Geometry: final body of the model. Coordinates: model frame, mm. Face numbers are marked on the shaded views. Coordinates: 2 decimals unless noted, no trailing zeros. Loops run counter-clockwise (first coordinate to the right, second up) from the corner with the lowest first, then second, coordinate; pieces in that order, holes last. Notation, with made-up numbers: (-24.5, -13.75) - (14.5, -13.75) arc R16 cw to (14.5, -3.75) - close; hole circle Ø9 at (75.25, 24.5). An arc over 180 degrees is marked (long way). Return JSON: item names as keys, results as strings.
from build123d import *

# Parameters (mm, degrees)
ESQUISSE1_W               = 58
ESQUISSE1_H               = 65
T_LE_DE_BASE_PLI_E1_DEPTH = 3
ENL_V_MAT_EXTRU_1_REACH   = 45.661
ESQUISSE6_R               = 2
ENL_V_MAT_EXTRU_2_REACH   = 45.661
ESQUISSE7_R               = 2
ESQUISSE8_R               = 4
ESQUISSE8_R_2             = 2
BOSS_EXTRU_1_DEPTH        = 2.7
ESQUISSE11_R              = 4
BOSS_EXTRU_3_DEPTH        = 1
ENL_V_MAT_EXTRU_3_REACH   = 46.07
ESQUISSE9_W               = 40
ESQUISSE9_H               = 34
ESQUISSE12_R              = 4
ESQUISSE12_R_2            = 2
BOSS_EXTRU_4_DEPTH        = 3.7
ESQUISSE13_R              = 2
BOSS_EXTRU_5_DEPTH        = 1


# Sheet-metal steps are written as plain solids
with BuildPart() as part:
    # Esquisse1 → Tôle de base pliée1 (new body)
    with BuildSketch(Plane.XY):
        Rectangle(ESQUISSE1_W, ESQUISSE1_H)
    extrude(amount=-T_LE_DE_BASE_PLI_E1_DEPTH)

    # Esquisse6 → Enlèv. mat.-Extru.1 (cut, up to next)
    with BuildSketch(Plane.XY, mode=Mode.PRIVATE) as enl_v_mat_extru_1_sk1:
        with Locations((-8.76, 28)):
            Circle(ESQUISSE6_R)
    enl_v_mat_extru_1_tool1 = extrude(enl_v_mat_extru_1_sk1.sketch, amount=-ENL_V_MAT_EXTRU_1_REACH, mode=Mode.PRIVATE) & part.part
    # Esquisse6 → Enlèv. mat.-Extru.1 (cut, up to next)
    with BuildSketch(Plane.XY, mode=Mode.PRIVATE) as enl_v_mat_extru_1_sk2:
        with Locations((19.18, 28)):
            Circle(ESQUISSE6_R)
    enl_v_mat_extru_1_tool2 = extrude(enl_v_mat_extru_1_sk2.sketch, amount=-ENL_V_MAT_EXTRU_1_REACH, mode=Mode.PRIVATE) & part.part
    # Esquisse6 → Enlèv. mat.-Extru.1 (cut, up to next)
    with BuildSketch(Plane.XY, mode=Mode.PRIVATE) as enl_v_mat_extru_1_sk3:
        with Locations((-24, -22.8)):
            Circle(ESQUISSE6_R)
    enl_v_mat_extru_1_tool3 = extrude(enl_v_mat_extru_1_sk3.sketch, amount=-ENL_V_MAT_EXTRU_1_REACH, mode=Mode.PRIVATE) & part.part
    # Esquisse6 → Enlèv. mat.-Extru.1 (cut, up to next)
    with BuildSketch(Plane.XY, mode=Mode.PRIVATE) as enl_v_mat_extru_1_sk4:
        with Locations((24.26, -24.07)):
            Circle(ESQUISSE6_R)
    enl_v_mat_extru_1_tool4 = extrude(enl_v_mat_extru_1_sk4.sketch, amount=-ENL_V_MAT_EXTRU_1_REACH, mode=Mode.PRIVATE) & part.part
    add(enl_v_mat_extru_1_tool1.solids().sort_by_distance((-8.76, 28, 0))[0], mode=Mode.SUBTRACT)
    add(enl_v_mat_extru_1_tool2.solids().sort_by_distance((19.18, 28, 0))[0], mode=Mode.SUBTRACT)
    add(enl_v_mat_extru_1_tool3.solids().sort_by_distance((-24, -22.8, 0))[0], mode=Mode.SUBTRACT)
    add(enl_v_mat_extru_1_tool4.solids().sort_by_distance((24.26, -24.07, 0))[0], mode=Mode.SUBTRACT)

    # Esquisse7 → Enlèv. mat.-Extru.2 (cut, up to next)
    with BuildSketch(Plane.XY, mode=Mode.PRIVATE) as enl_v_mat_extru_2_sk1:
        with Locations((-17, -26.25)):
            Circle(ESQUISSE7_R)
    enl_v_mat_extru_2_tool1 = extrude(enl_v_mat_extru_2_sk1.sketch, amount=-ENL_V_MAT_EXTRU_2_REACH, mode=Mode.PRIVATE) & part.part
    # Esquisse7 → Enlèv. mat.-Extru.2 (cut, up to next)
    with BuildSketch(Plane.XY, mode=Mode.PRIVATE) as enl_v_mat_extru_2_sk2:
        with Locations((0, -26.25)):
            Circle(ESQUISSE7_R)
    enl_v_mat_extru_2_tool2 = extrude(enl_v_mat_extru_2_sk2.sketch, amount=-ENL_V_MAT_EXTRU_2_REACH, mode=Mode.PRIVATE) & part.part
    # Esquisse7 → Enlèv. mat.-Extru.2 (cut, up to next)
    with BuildSketch(Plane.XY, mode=Mode.PRIVATE) as enl_v_mat_extru_2_sk3:
        with Locations((17, -26.25)):
            Circle(ESQUISSE7_R)
    enl_v_mat_extru_2_tool3 = extrude(enl_v_mat_extru_2_sk3.sketch, amount=-ENL_V_MAT_EXTRU_2_REACH, mode=Mode.PRIVATE) & part.part
    # Esquisse7 → Enlèv. mat.-Extru.2 (cut, up to next)
    with BuildSketch(Plane.XY, mode=Mode.PRIVATE) as enl_v_mat_extru_2_sk4:
        with Locations((0, 21.25)):
            Circle(ESQUISSE7_R)
    enl_v_mat_extru_2_tool4 = extrude(enl_v_mat_extru_2_sk4.sketch, amount=-ENL_V_MAT_EXTRU_2_REACH, mode=Mode.PRIVATE) & part.part
    # Esquisse7 → Enlèv. mat.-Extru.2 (cut, up to next)
    with BuildSketch(Plane.XY, mode=Mode.PRIVATE) as enl_v_mat_extru_2_sk5:
        with Locations((17, 21.25)):
            Circle(ESQUISSE7_R)
    enl_v_mat_extru_2_tool5 = extrude(enl_v_mat_extru_2_sk5.sketch, amount=-ENL_V_MAT_EXTRU_2_REACH, mode=Mode.PRIVATE) & part.part
    # Esquisse7 → Enlèv. mat.-Extru.2 (cut, up to next)
    with BuildSketch(Plane.XY, mode=Mode.PRIVATE) as enl_v_mat_extru_2_sk6:
        with Locations((-17, 21.25)):
            Circle(ESQUISSE7_R)
    enl_v_mat_extru_2_tool6 = extrude(enl_v_mat_extru_2_sk6.sketch, amount=-ENL_V_MAT_EXTRU_2_REACH, mode=Mode.PRIVATE) & part.part
    add(enl_v_mat_extru_2_tool1.solids().sort_by_distance((-17, -26.25, 0))[0], mode=Mode.SUBTRACT)
    add(enl_v_mat_extru_2_tool2.solids().sort_by_distance((0, -26.25, 0))[0], mode=Mode.SUBTRACT)
    add(enl_v_mat_extru_2_tool3.solids().sort_by_distance((17, -26.25, 0))[0], mode=Mode.SUBTRACT)
    add(enl_v_mat_extru_2_tool4.solids().sort_by_distance((0, 21.25, 0))[0], mode=Mode.SUBTRACT)
    add(enl_v_mat_extru_2_tool5.solids().sort_by_distance((17, 21.25, 0))[0], mode=Mode.SUBTRACT)
    add(enl_v_mat_extru_2_tool6.solids().sort_by_distance((-17, 21.25, 0))[0], mode=Mode.SUBTRACT)

    # Esquisse8 → Boss.-Extru.1 (add)
    # profile 1 of 4: a face of its own
    with BuildSketch(Plane.XY.offset(-3)):
        with Locations((-8.76, 28)):
            Circle(ESQUISSE8_R)
        with Locations((-8.76, 28)):
            Circle(ESQUISSE8_R_2, mode=Mode.SUBTRACT)
    # profile 2 of 4: a face of its own
    with BuildSketch(Plane.XY.offset(-3)):
        with Locations((19.18, 28)):
            Circle(ESQUISSE8_R)
        with Locations((19.18, 28)):
            Circle(ESQUISSE8_R_2, mode=Mode.SUBTRACT)
    # profile 3 of 4: a face of its own
    with BuildSketch(Plane.XY.offset(-3)):
        with Locations((24.26, -24.07)):
            Circle(ESQUISSE8_R)
        with Locations((24.26, -24.07)):
            Circle(ESQUISSE8_R_2, mode=Mode.SUBTRACT)
    # profile 4 of 4: a face of its own
    with BuildSketch(Plane.XY.offset(-3)):
        with Locations((-24, -22.8)):
            Circle(ESQUISSE8_R)
        with Locations((-24, -22.8)):
            Circle(ESQUISSE8_R_2, mode=Mode.SUBTRACT)
    extrude(amount=-BOSS_EXTRU_1_DEPTH)

    # Esquisse11 → Boss.-Extru.3 (add)
    with BuildSketch(Plane(origin=(0, 0, -5.7), x_dir=(-1, 0, 0), z_dir=(0, 0, -1))):
        with Locations(Location((24, -22.8, 0), (0, 0, 180))):
            Circle(ESQUISSE11_R)
        with Locations(Location((8.76, 28, 0), (0, 0, 180))):
            Circle(ESQUISSE11_R)
        with Locations(Location((-24.26, -24.07, 0), (0, 0, 180))):
            Circle(ESQUISSE11_R)
        with Locations(Location((-19.18, 28, 0), (0, 0, 180))):
            Circle(ESQUISSE11_R)
    extrude(amount=BOSS_EXTRU_3_DEPTH)

    # Esquisse9 → Enlèv. mat.-Extru.3 (cut, up to next)
    with BuildSketch(Plane.XY, mode=Mode.PRIVATE) as enl_v_mat_extru_3_sk1:
        Rectangle(ESQUISSE9_W, ESQUISSE9_H)
    enl_v_mat_extru_3_tool1 = extrude(enl_v_mat_extru_3_sk1.sketch, amount=-ENL_V_MAT_EXTRU_3_REACH, mode=Mode.PRIVATE) & part.part
    add(enl_v_mat_extru_3_tool1.solids().sort_by_distance((0, 0, 0))[0], mode=Mode.SUBTRACT)

    # Esquisse12 → Boss.-Extru.4 (add)
    # profile 1 of 6: a face of its own
    with BuildSketch(Plane(origin=(0, 0, -3), x_dir=(-1, 0, 0), z_dir=(0, 0, -1))):
        with Locations((-17, 21.25)):
            Circle(ESQUISSE12_R)
        with Locations(Location((-17, 21.25, 0), (0, 0, 180))):
            Circle(ESQUISSE12_R_2, mode=Mode.SUBTRACT)
    # profile 2 of 6: a face of its own
    with BuildSketch(Plane(origin=(0, 0, -3), x_dir=(-1, 0, 0), z_dir=(0, 0, -1))):
        with Locations(Location((0, 21.25, 0), (0, 0, 180))):
            Circle(ESQUISSE12_R)
        with Locations(Location((0, 21.25, 0), (0, 0, 180))):
            Circle(ESQUISSE12_R_2, mode=Mode.SUBTRACT)
    # profile 3 of 6: a face of its own
    with BuildSketch(Plane(origin=(0, 0, -3), x_dir=(-1, 0, 0), z_dir=(0, 0, -1))):
        with Locations(Location((17, 21.25, 0), (0, 0, 180))):
            Circle(ESQUISSE12_R)
        with Locations(Location((17, 21.25, 0), (0, 0, 180))):
            Circle(ESQUISSE12_R_2, mode=Mode.SUBTRACT)
    # profile 4 of 6: a face of its own
    with BuildSketch(Plane(origin=(0, 0, -3), x_dir=(-1, 0, 0), z_dir=(0, 0, -1))):
        with Locations((17, -26.25)):
            Circle(ESQUISSE12_R)
        with Locations(Location((17, -26.25, 0), (0, 0, 180))):
            Circle(ESQUISSE12_R_2, mode=Mode.SUBTRACT)
    # profile 5 of 6: a face of its own
    with BuildSketch(Plane(origin=(0, 0, -3), x_dir=(-1, 0, 0), z_dir=(0, 0, -1))):
        with Locations(Location((0, -26.25, 0), (0, 0, 180))):
            Circle(ESQUISSE12_R)
        with Locations(Location((0, -26.25, 0), (0, 0, 180))):
            Circle(ESQUISSE12_R_2, mode=Mode.SUBTRACT)
    # profile 6 of 6: a face of its own
    with BuildSketch(Plane(origin=(0, 0, -3), x_dir=(-1, 0, 0), z_dir=(0, 0, -1))):
        with Locations((-17, -26.25)):
            Circle(ESQUISSE12_R)
        with Locations(Location((-17, -26.25, 0), (0, 0, 180))):
            Circle(ESQUISSE12_R_2, mode=Mode.SUBTRACT)
    extrude(amount=BOSS_EXTRU_4_DEPTH)

    # Esquisse13 → Boss.-Extru.5 (add)
    with BuildSketch(Plane.XY):
        with Locations((-17, 21.25)):
            Circle(ESQUISSE13_R)
        with Locations((-17, -26.25)):
            Circle(ESQUISSE13_R)
        with Locations((0, 21.25)):
            Circle(ESQUISSE13_R)
        with Locations((0, -26.25)):
            Circle(ESQUISSE13_R)
        with Locations((17, -26.25)):
            Circle(ESQUISSE13_R)
        with Locations((17, 21.25)):
            Circle(ESQUISSE13_R)
    extrude(amount=-BOSS_EXTRU_5_DEPTH)


solid = part.part
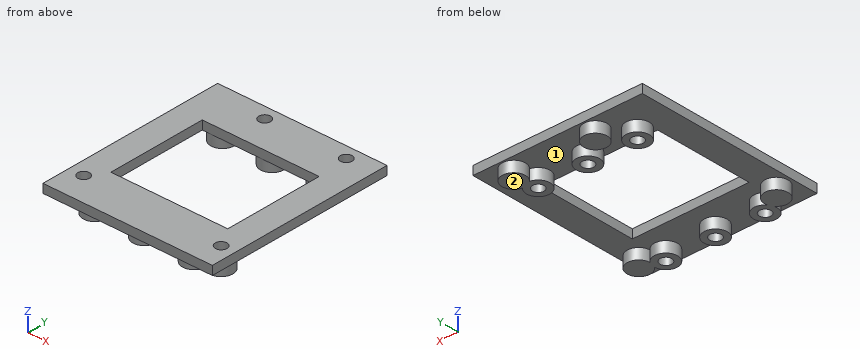
Item 1: Ray query, probe 1 along Y at (x, z) = (19.18, -2.9); probe 2 along X at (y, z) = (-26.25, -2.2); probe 3 along Y at (x, z) = (-8.76, -3.25). Return the intervals inside material, ascending. Write a range as from..to.
Worked out:
{"probe 1": "-32.5..-17, 17..26, 30..32.5", "probe 2": "-29..-19, -15..-2, 2..15, 19..29", "probe 3": "24..26, 30..32"}
Item 2: Mould query, pull axis X, two halves, no side actions, for the marked faces 1 and 2. Classes: +X half, -X half, draft (parallel to the pull), parting line (faces both ways), or undercut.
Worked out:
{"face 1": "undercut", "face 2": "draft"}
Item 3: Section query B-B, the plane z = -3.75. Count the separate pieces of the cut face and the enclosed holes in it, and give its area (3 significant figures).
Worked out:
{"separate pieces": "7", "enclosed holes": "10", "area": "374 mm^2"}
Item 4: Section query C-C, the plane x = 0. Return loops of the section in (y, z).
Worked out:
{"outline": "(-32.5, -3) - (-30.25, -3) - (-30.25, -6.7) - (-28.25, -6.7) - (-28.25, -1) - (-24.25, -1) - (-24.25, -6.7) - (-22.25, -6.7) - (-22.25, -3) - (-17, -3) - (-17, 0) - (-32.5, 0) - close; (17, -3) - (17.25, -3) - (17.25, -6.7) - (19.25, -6.7) - (19.25, -1) - (23.25, -1) - (23.25, -6.7) - (25.25, -6.7) - (25.25, -3) - (32.5, -3) - (32.5, 0) - (17, 0) - close"}
Item 5: Section query D-D, the plane y = 28. Return loops of the section in (x, z), and give its area (3 significant figures).
Worked out:
{"outline": "(-29, -3) - (-12.76, -3) - (-12.76, -6.7) - (-4.76, -6.7) - (-4.76, -3) - (15.18, -3) - (15.18, -6.7) - (23.18, -6.7) - (23.18, -3) - (29, -3) - (29, 0) - (21.18, 0) - (21.18, -5.7) - (17.18, -5.7) - (17.18, 0) - (-6.76, 0) - (-6.76, -5.7) - (-10.76, -5.7) - (-10.76, 0) - (-29, 0) - close", "area": "188 mm^2"}
Item 6: First-contact query: pin 1 Ø1 at (y, z) = (-22, -5) entering from +X; pin 2 Ø2 at (x, y) = (17, -27) entering from -Z; pin 3 Ø1.5 at (y, z) = (-19, -5.5) entering from +X. Flat tips, straight axial feed; report the tip coordinate or a pass-through.
Worked out:
{"pin 1": "x = 27.94", "pin 2": "z = -1", "pin 3": "x = -21.41"}
Item 7: Section query A-A, the plane y = 16. Return loops of the section in (x, z).
Worked out:
{"outline": "(-29, -3) - (-20, -3) - (-20, 0) - (-29, 0) - close; (20, -3) - (29, -3) - (29, 0) - (20, 0) - close"}
